Answer from the drawing. Dimensions are ordinates in mm from the lowest x, y and z of the part. Coordinates: 2 decimals unless noted, no trailing zeros. Order: outer loops, then holes, each group sorted by start corner. A loop starts at its lowest first (then second) coordinate and runs counter-clockwise, first axis right, second up. Notation, with made-up numbers: (-20, 12) -> (33, 12) arc R10 ccw to (33, 25) -> close; hole circle Ø4 at (67, -26). An arc over 180 degrees is marked (long way). Answer in a Markdown table with one row per item.
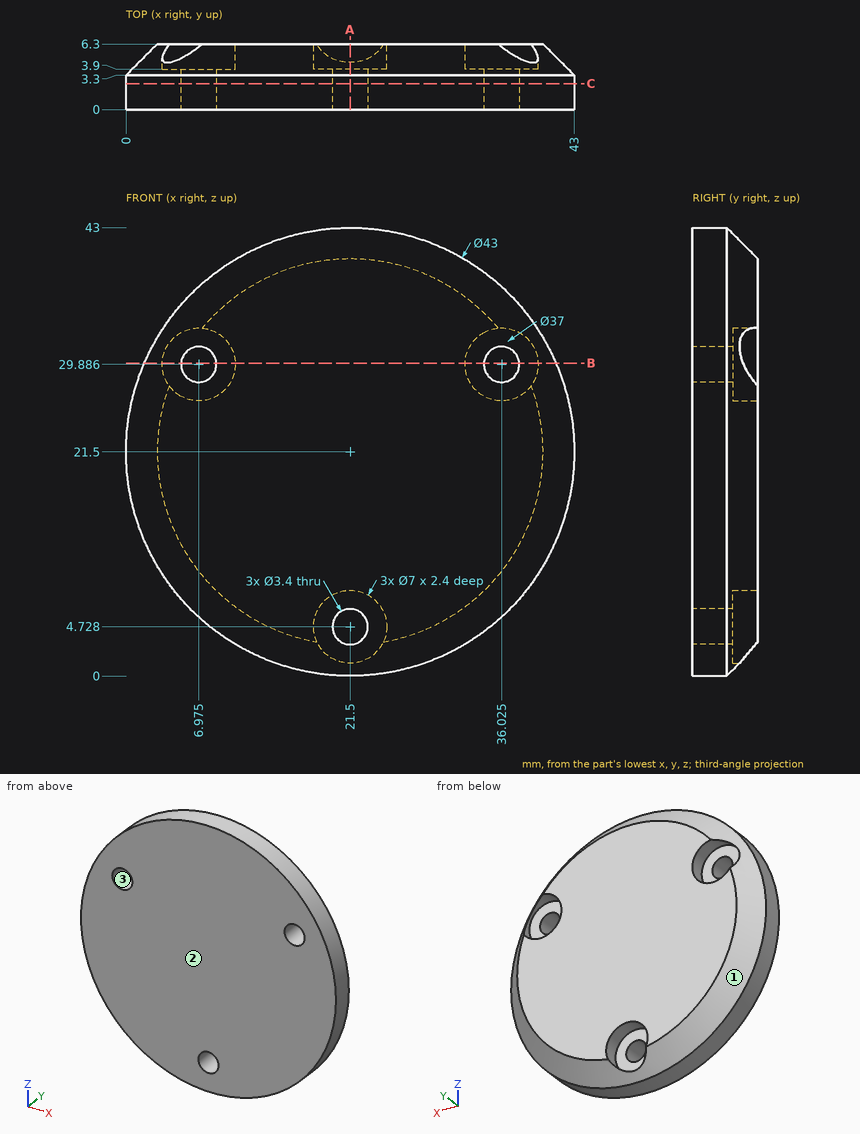
(1) A cutting plane is placed at C-C, the plane y = 2.5. Determine the outline of the cut face in (x, z) (1 decimal).
Check values:
| item | result |
|---|---|
| outline | circle Ø43 at (21.5, 21.5); hole circle Ø3.4 at (7, 29.9); hole circle Ø3.4 at (21.5, 4.7); hole circle Ø3.4 at (36, 29.9) |
(2) A cutting plane is placed at A-A, the plane x = 21.5. Determine the outline of the cut face in (y, z).
Check values:
| item | result |
|---|---|
| outline | (0, 0) -> (3.3, 0) -> (4.53, 1.23) -> (3.9, 1.23) -> (3.9, 3.03) -> (0, 3.03) -> close; (0, 6.43) -> (3.9, 6.43) -> (3.9, 8.23) -> (6.3, 8.23) -> (6.3, 40) -> (3.3, 43) -> (0, 43) -> close |
(3) For a pull along X with two mould halves and no side action, classify the marked faces 1, 2 and 3 as released by +X, released by -X, zero draft, split by the parting line, or undercut.
Check values:
| item | result |
|---|---|
| face 1 | split by the parting line |
| face 2 | zero draft |
| face 3 | undercut |
(4) Find the intervals of material crossed by line 1 along X through (y, z) = (1.5, 22); line 2 along Z through (x, y) = (18.5, 4.75) (1 decimal); line 3 along X through (y, z) = (4.25, 31), in increasing order. Write a range as from..to.
Check values:
| item | result |
|---|---|
| line 1 | 0.01..42.99 |
| line 2 | 1.7..2.9, 6.5..41.3 |
| line 3 | 3.28..3.66, 10.29..32.71, 39.34..39.72 |
(5) Flat-ended cylindrical pins translate along their axes: pin 1 (4 mm diameter, centred on x = 21.5, z = 4.73, fed in from +Y); pin 2 (3 mm diameter, centred on y = 5.5, z = 34, fed in from -X); pin 3 (3 mm diameter, centred on x = 36.03, z = 29.89, fed in from -Y) (3 decimals). Find the tip coordinate at first contact, or state that the pin passes through.
Check values:
| item | result |
|---|---|
| pin 1 | y = 3.9 |
| pin 2 | x = 4.58 |
| pin 3 | through |
(6) A cutting plane is placed at B-B, the plane z = 30. Count the separate pieces of the cut face and the enclosed holes in it, then the cut area to 3 significant figures.
Check values:
| item | result |
|---|---|
| separate pieces | 3 |
| enclosed holes | 0 |
| area | 181 mm² |
